CAD build for the part. Positions are in the model's coordinates, mm. Face numbers are marked on the shaded views. A direction names the side the tool comes from. Coordinates: 2 decimals unless noted, no trailing zeros. Order: outer loops, then holes, each group sorted by start corner. A loop starts at its lowest first (then second) coordinate and runs counter-clockwise, first axis right, second up. Notation, with made-up numbers: (-26, 78) - (8, 78) arc R20 cw to (8, 83) - close; hole circle Ø8 at (-8, 64.5). An arc over 180 degrees is marked (long way). Write each question's results on one line, items separated by ' | '. Start each with the question number.
Q1. Which spindle directions (+Z, -Z, +X, -X, +Y, -Y) get a long thin tool onto all of the face, cutting with end or side? Do the marked faces 4, 5 and 6. Say none if no direction does.
Q2. Band-saw the part on D-D, the plane z = -3. Write the cut outline in (x, y), then the cut area to 3 significant figures.
Q3. Band-saw the part on A-A, the plane x = 0. Write the cut outline in (y, z).
Q4. Band-saw the part on B-B, the plane x = -4.25. Write the cut outline in (y, z).
Q5. Wall check: probe 1 along Z at (x, y) = (-4.75, 0); probe 2 along Z at (x, y) = (7.1, 0); probe 3 along X at (y, z) = (-2, -21). Give the ranges that are in metal, low to high.
Q6. Pin check, flat tips, straight feed: P1, Ø5, axis at x = -1, y = 11.5, coming from the +Z side; P2, Ø3, axis at x = 1.5, y = 6, coming from the +Z side; P3, Ø6, axis at x = -4.5, z = 16.5, coming from the +Y side; P4, Ø2, axis at x = 0, y = 11.25, coming from the +Z side. Stop position of each tip, or through.
Q7. Band-saw the part on C-C, the plane z = 17.5. Write the cut outline in (x, y).
Q8. Pull direction X, two halves, no side cores. Call the marked faces 1, 2 and 3: released by +X, released by -X, zero draft, split by the parting line, or undercut.
```python
from build123d import *

# Parameters (mm, degrees)
F0_W      = 6.5
F0_H      = 7.5
F1_DEPTH  = 8
F3_DEPTH  = 2
F4_DEPTH  = 25
F6_DEPTH  = 2
F7_R      = 5
F8_R      = 5
F9_R      = 1
F10_DEPTH = 14.5
F11_R     = 1.25
F12_DEPTH = 32.501
F13_R     = 2.5
F14_R     = 1.25
F15_DEPTH = 32.501
F17_DEPTH = 1


with BuildPart() as f1:
    # F0 (on Front) → F1 (new body, symmetric)
    with BuildSketch(Plane.XZ):
        Polygon((3.5, -28.75), (8, -28.75), (8, 28.75), (3.5, 28.75), (3.5, 18.75), (-3.5, 18.75), (-3.5, 28.75), (-8, 28.75), (-8, -28.75), (-3.5, -28.75), (-3.5, -18.75), (3.5, -18.75), align=None)
        Rectangle(F0_W, F0_H, mode=Mode.SUBTRACT)
    extrude(amount=F1_DEPTH, both=True)

    # F2 (on face) → F3 (cut)
    with BuildSketch(Plane.YZ.offset(8)):
        with BuildLine():
            ThreePointArc((2.75, 24.5), (1.9445436483, 26.4445436483), (0, 27.25))
            ThreePointArc((0, 27.25), (-1.9445436483, 22.5554563517), (2.75, 24.5))
        make_face()
        with BuildLine():
            ThreePointArc((1.5, 24.5), (-1.0606601718, 23.4393398282), (0, 26))
            ThreePointArc((0, 26), (1.0606601718, 25.5606601718), (1.5, 24.5))
        make_face(mode=Mode.SUBTRACT)
        with BuildLine():
            ThreePointArc((2.75, -24.5), (-1.9445436483, -22.5554563517), (0, -27.25))
            ThreePointArc((0, -27.25), (1.9445436483, -26.4445436483), (2.75, -24.5))
        make_face()
        with BuildLine():
            ThreePointArc((1.5, -24.5), (1.0606601718, -25.5606601718), (0, -26))
            ThreePointArc((0, -26), (-1.0606601718, -23.4393398282), (1.5, -24.5))
        make_face(mode=Mode.SUBTRACT)
    extrude(amount=-F3_DEPTH, mode=Mode.SUBTRACT)

    # F4 (cut): faces of the model
    f4_faces = [f1.faces().sort_by_distance(p)[0] for p in [
        (8, 0, 24.5),
        (8, 0, -24.5),
    ]]
    extrude(f4_faces, amount=-F4_DEPTH, mode=Mode.SUBTRACT)

    # F5 (on face) → F6 (cut)
    with BuildSketch(Plane(origin=(-8, 0, 0), x_dir=(0, -1, 0), z_dir=(-1, 0, 0))):
        Polygon((1.4860554785, 27.1748780249), (0, 27.1503606325), (-1.5734845824, 27.1244008083), (-3.0595400608, 24.4495227834), (-1.4860554785, 21.8251219751), (1.5734845824, 21.8755991917), (3.0595400608, 24.5504772166), align=None)
        with BuildLine():
            ThreePointArc((1.5, 24.5), (-1.0606601718, 23.4393398282), (0, 26))
            ThreePointArc((0, 26), (1.0606601718, 25.5606601718), (1.5, 24.5))
        make_face(mode=Mode.SUBTRACT)
        Polygon((-1.4958462814, -27.1694151487), (0, -27.1502182166), (1.5638581913, -27.1301484541), (3.0597044727, -24.4607333055), (1.4958462814, -21.8305848513), (-1.5638581913, -21.8698515459), (-3.0597044727, -24.5392666945), align=None)
        with BuildLine():
            ThreePointArc((1.5, -24.5), (1.0606601718, -25.5606601718), (0, -26))
            ThreePointArc((0, -26), (-1.0606601718, -23.4393398282), (1.5, -24.5))
        make_face(mode=Mode.SUBTRACT)
    extrude(amount=-F6_DEPTH, mode=Mode.SUBTRACT)

    # F7
    f7_edges = [f1.edges().sort_by_distance(p)[0] for p in [
        (5.75, -8, 28.75),
        (5.75, 8, 28.75),
        (-5.75, 8, 28.75),
        (-5.75, -8, 28.75),
    ]]
    fillet(f7_edges, radius=F7_R)

    # F8
    f8_edges = [f1.edges().sort_by_distance(p)[0] for p in [
        (5.75, 8, -28.75),
        (-5.75, 8, -28.75),
        (5.75, -8, -28.75),
        (-5.75, -8, -28.75),
    ]]
    fillet(f8_edges, radius=F8_R)

    # F9
    f9_edges = [f1.edges().sort_by_distance(p)[0] for p in [
        (-8, -8, 0),
        (8, -8, 0),
        (8, 8, 0),
        (-8, 8, 0),
    ]]
    fillet(f9_edges, radius=F9_R)

    # F0 (on Front) → F10 (join, symmetric)
    with BuildSketch(Plane.XZ):
        Rectangle(F0_W, F0_H)
    extrude(amount=F10_DEPTH, both=True)

    # F11 (on face) → F12 (cut, through all)
    with BuildSketch(Plane.XY.offset(3.75)):
        with Locations((0, 11.25)):
            Circle(F11_R)
        with Locations((0, -11.25)):
            Circle(F11_R)
    extrude(amount=-F12_DEPTH, mode=Mode.SUBTRACT)

    # F13
    f13_edges = [f1.edges().sort_by_distance(p)[0] for p in [
        (-3.25, 14.5, 0),
        (3.25, 14.5, 0),
        (-3.25, -14.5, 0),
        (3.25, -14.5, 0),
    ]]
    fillet(f13_edges, radius=F13_R)

    # F14 (on face) → F15 (cut, through all)
    with BuildSketch(Plane.XY.offset(3.75)):
        with BuildLine():
            ThreePointArc((-3.25, -12), (-2.517766953, -13.767766953), (-0.75, -14.5))
            Line((-0.75, -14.5), (0.75, -14.5))
            ThreePointArc((0.75, -14.5), (2.517766953, -13.767766953), (3.25, -12))
            Line((3.25, -12), (3.25, -8))
            Line((3.25, -8), (-3.25, -8))
            Line((-3.25, -8), (-3.25, -12))
        make_face()
        with Locations((0, -11.25)):
            Circle(F14_R, mode=Mode.SUBTRACT)
    extrude(amount=-F15_DEPTH, mode=Mode.SUBTRACT)

    # F16 (on Right) → F17 (cut, symmetric)
    with BuildSketch(Plane.YZ):
        with BuildLine():
            ThreePointArc((-8, -8), (-4, 0), (-8, 8))
            Line((-8, 8), (-8, 5.2915026221))
            ThreePointArc((-8, 5.2915026221), (-6, 0), (-8, -5.2915026221))
            Line((-8, -5.2915026221), (-8, -8))
        make_face()
    extrude(amount=F17_DEPTH, both=True, mode=Mode.SUBTRACT)


solid = f1.part
```
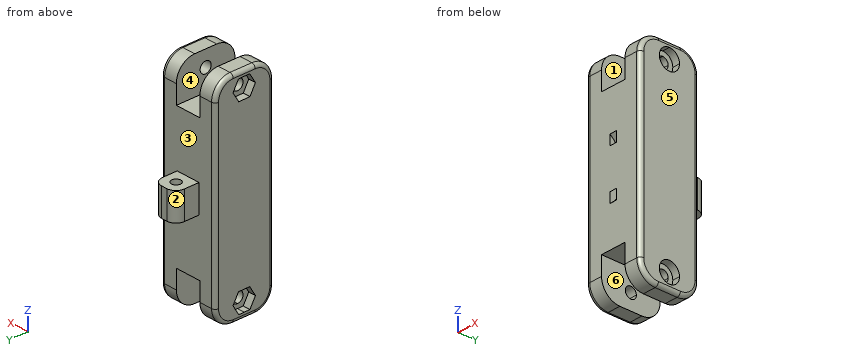
Results below:
1) face 4: +Z, +Y, -Y | face 5: +Z, -Z, +X, +Y, -Y | face 6: -Z, +Y, -Y
2) outline: (-8, -7) arc R1 ccw to (-7, -8) - (7, -8) arc R1 ccw to (8, -7) - (8, 7) arc R1 ccw to (7, 8) - (3.25, 8) - (3.25, 12) arc R2.5 ccw to (0.75, 14.5) - (-0.75, 14.5) arc R2.5 ccw to (-3.25, 12) - (-3.25, 8) - (-7, 8) arc R1 ccw to (-8, 7) - close; hole circle Ø2.5 at (0, 11.25); hole (-1, -6.58) - (1, -6.58) - (1, -4.46) - (-1, -4.46) - close | area: 286 mm²
3) outline: (-8, -18.75) - (8, -18.75) - (8, -3.75) - (10, -3.75) - (10, 3.75) - (8, 3.75) - (8, 18.75) - (-8, 18.75) - (-8, 8) arc R10 cw to (-8, -8) - close; (-8, -5.29) arc R8 ccw to (-8, 5.29) - close; (12.5, -3.75) - (14.5, -3.75) - (14.5, 3.75) - (12.5, 3.75) - close
4) outline: (-8, -23.75) arc R5 ccw to (-3, -28.75) - (3, -28.75) arc R5 ccw to (8, -23.75) - (8, 23.75) arc R5 ccw to (3, 28.75) - (-3, 28.75) arc R5 ccw to (-8, 23.75) - close; hole circle Ø3 at (0, -24.5); hole circle Ø3 at (0, 24.5)
5) probe 1: z = -28.75 to -26, -23 to 23, 26 to 28.75 | probe 2: z = -28.74 to -27.25, -21.75 to 21.75, 27.25 to 28.74 | probe 3: x = -8 to -3.5, 3.5 to 8
6) P1: stops at z = 3.75 | P2: stops at z = 18.75 | P3: stops at y = 8 | P4: passes through
7) outline: (-8, -7) arc R1 ccw to (-7, -8) - (7, -8) arc R1 ccw to (8, -7) - (8, 7) arc R1 ccw to (7, 8) - (-7, 8) arc R1 ccw to (-8, 7) - close
8) face 1: undercut | face 2: released by -X | face 3: zero draft
